The model under review builds one solid part; all positions refer to its coordinate system, in mm. A direction names the side the tool comes from. Round coordinates to 2 decimals unless told otherwise and drop trailing zeros. Order: outer loops, then holes, each group sorted by start corner. A loop starts at its lowest first (then second) coordinate and runs counter-clockwise, first axis right, second up.
```python
from build123d import *

# Parameters (mm, degrees)
ESBO_O1_R                  = 12.5
ESBO_O1_R_2                = 10
RESSALTO_EXTRUS_O1_DEPTH   = 130
CORTE_EXTRUS_O1_DEPTH      = 5
CORTE_EXTRUS_O1_DEPTH_BACK = 5
ESBO_O2_R                  = 12.5
ESBO_O2_R_2                = 12


with BuildPart() as part:
    # Esboço1 → Ressalto-extrusão1 (new body)
    with BuildSketch(Plane.XY):
        Circle(ESBO_O1_R)
        Circle(ESBO_O1_R_2, mode=Mode.SUBTRACT)
    extrude(amount=RESSALTO_EXTRUS_O1_DEPTH)

    # Esboço2 → Corte-extrusão1 (cut, two sides: drawn at the far end of the back side and taken through both)
    with BuildSketch(Plane(origin=(0, 0, 0), x_dir=(0, 0, -1), z_dir=(1, 0, 0)).offset(-CORTE_EXTRUS_O1_DEPTH_BACK)):
        with Locations((5, 0)):
            Circle(ESBO_O2_R)
        with Locations((5, 0)):
            Circle(ESBO_O2_R_2, mode=Mode.SUBTRACT)
    extrude(amount=CORTE_EXTRUS_O1_DEPTH + CORTE_EXTRUS_O1_DEPTH_BACK, mode=Mode.SUBTRACT)


solid = part.part
```
(1) For faces 4 (the flat face through (-5, 10, 2)), 5 (the cylindrical face through (-2.17, -9.76, 64.09)), list the 3-axis set-ups (+Z, -Z, +X, -X, +Y, -Y) from which the entire face can be reached by the end or side of a thin tool; tool diameter is ignored.
Data:
face 4: none
face 5: +Z, -Z
(2) Consider section D-D (x = 8.25). Write out the cut boundary in (y, z).
Data:
outline: (-9.39, 0) - (-5.65, 0) - (-5.65, 130) - (-9.39, 130) - close; (5.65, 0) - (9.39, 0) - (9.39, 130) - (5.65, 130) - close
(3) To check wall thickness, follow probe 1 along Y at (x, z) = (0, 60); probe 2 along X at (y, z) = (5, 36.5). State the ranges of each line that lie inside material, in increasing order.
Data:
probe 1: y = -12.5 to -10, 10 to 12.5
probe 2: x = -11.46 to -8.66, 8.66 to 11.46
(4) Consider section A-A (y = 0). Write out the cut boundary in (x, z), and give its area (3 significant figures).
Data:
outline: (-12.5, 0) - (-10, 0) - (-10, 130) - (-12.5, 130) - close; (10, 0) - (12.5, 0) - (12.5, 130) - (10, 130) - close
area: 650 mm2
(5) Draft analysis for pull direction Y (two halves, no side actions). For faces 1 (the cylindrical face through (-0.07, -10.38, 1.02)), 2 (the flat face through (-0.1, 10.2, 130)), 3 (the cylindrical face through (11.923, 3.755, 64.09)), state which applies: pulls with the +Y half, pulls with the -Y half, needs draft (parallel to the pull), parting line crosses it, or undercut.
Data:
face 1: undercut
face 2: needs draft
face 3: parting line crosses it
(6) Consider section C-C (z = 51). Write out the cut boundary in (x, y).
Data:
outline: circle Ø25 at (0, 0); hole circle Ø20 at (0, 0)
(7) Consider section B-B (x = 0). Write out the cut boundary in (y, z), and give its area (3 significant figures).
Data:
outline: (-12.5, 0) - (-11.46, 0) arc R12.5 cw to (-10, 2.5) - (-10, 130) - (-12.5, 130) - close; (-10.91, 0) - (-10, 0) - (-10, 1.63) arc R12 ccw to start; (10, 0) - (10.91, 0) arc R12 ccw to (10, 1.63) - close; (10, 2.5) arc R12.5 cw to (11.46, 0) - (12.5, 0) - (12.5, 130) - (10, 130) - close
area: 648 mm2
(8) Insertion check: pin 1 (0.8 mm diameter, centred on y = -10.5, z = 2.5, fed in from -X); pin 2 (3 mm diameter, centred on x = 9, z = 19, fed in from +Y); pin 3 (1.5 mm diameter, centred on y = -10, z = 71.5, fed in from +X); pin 4 (12 mm diameter, centred on x = 4, z = 107.5, fed in from +Y). Each pin has a flat end and moves straight along its axis. Give the tip position at first contact, or say it passes through.
Data:
pin 1: stops at x = -7.36
pin 2: stops at y = 10
pin 3: stops at x = 8.41
pin 4: stops at y = 12.5
